Design review of the part shown in the three views and the two pictorial views. Dimensions are in mm from the part's minimum x, y and z. Coordinates: 2 decimals unless noted, no trailing zeros. Loops run counter-clockwise (first coordinate to the right, second up) from the corner with the lowest first, then second, coordinate; pieces in that order, holes last. Notation, with made-up numbers: (68.5, -29) - (101.5, -29) arc R12 ccw to (101.5, -22) - close; hole circle Ø7 at (45.5, 74). An arc over 180 degrees is marked (long way). One line per item, written item: value. Start each with the question number.
1. Take a section at B-B, the plane z = 7. State the section outline as (x, y) points.
2. Take a section at D-D, the plane x = 38. State the section outline as (y, z) points, and give its area (3 significant figures).
3. To check wall thickness, follow line 1 (Z direction, x = 43.5, y = 13.75); line 2 (X direction, y = 6.5, z = 38.5); line 3 (Y direction, x = 23.5, z = 19). State the ranges of each line that lie inside material, in increasing order. Write a range as from..to.
4. The part is to be moulded in two halves that separate along X. For the marked faces 1, 2 and 3, say which applies: released by +X, released by -X, zero draft, split by the parting line, or undercut.
5. Insertion check: pin 1 (4 mm diameter, centred on y = 7.5, z = 40, fed in from -X); pin 2 (4 mm diameter, centred on x = 30.5, z = 35, fed in from -Y); pin 3 (3 mm diameter, centred on y = 4.5, z = 31.5, fed in from +X); pin 4 (5.5 mm diameter, centred on x = 37.5, y = 3.5, fed in from -Z). Each pin has a flat end and moves straight along its axis. Give the tip position at first contact, or say it passes through.
6. Take a section at C-C, the plane x = 15. State the section outline as (y, z) points, and give its area (3 significant figures).
7. Take a section at A-A, the plane y = 5. State the section outline as (x, z) points.
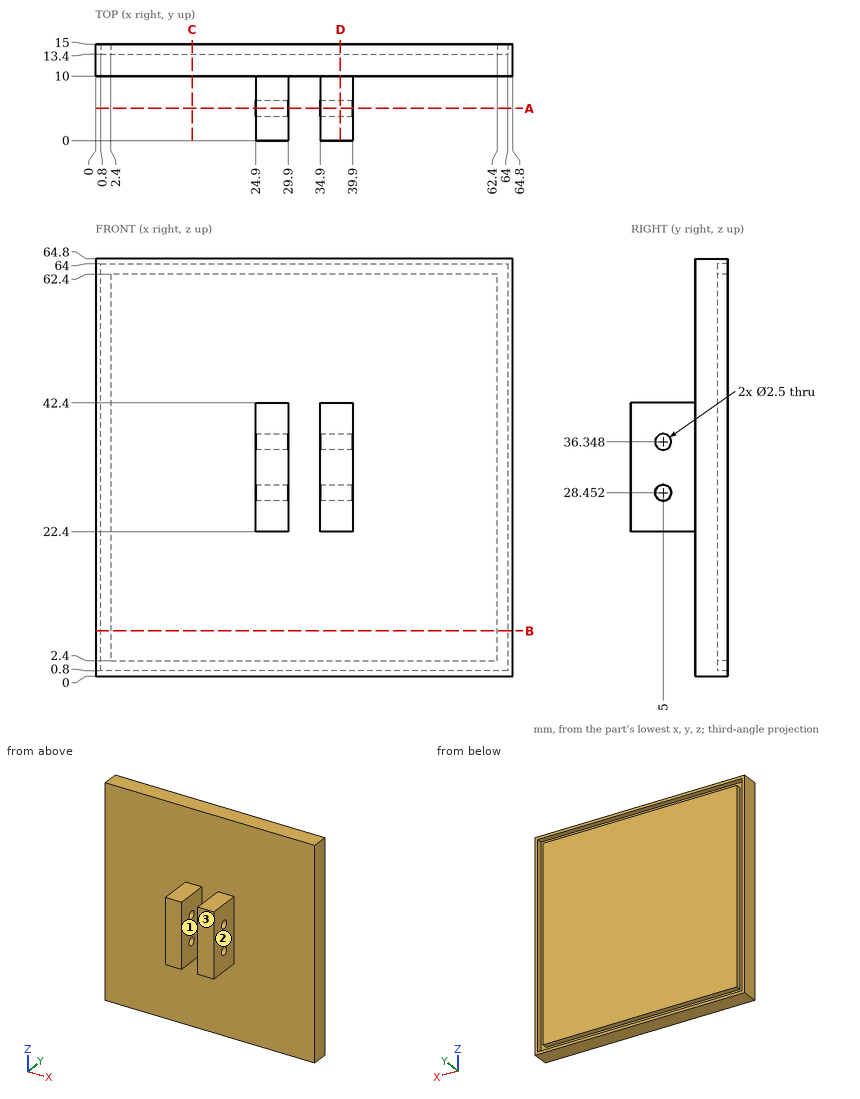
Solutions:
1. outline: (0, 10) - (64.8, 10) - (64.8, 15) - (64, 15) - (64, 13.4) - (62.4, 13.4) - (62.4, 15) - (2.4, 15) - (2.4, 13.4) - (0.8, 13.4) - (0.8, 15) - (0, 15) - close
2. outline: (0, 22.4) - (10, 22.4) - (10, 0) - (15, 0) - (15, 0.8) - (13.4, 0.8) - (13.4, 2.4) - (15, 2.4) - (15, 62.4) - (13.4, 62.4) - (13.4, 64) - (15, 64) - (15, 64.8) - (10, 64.8) - (10, 42.4) - (0, 42.4) - close; hole circle Ø2.5 at (5, 28.45); hole circle Ø2.5 at (5, 36.35)
2. area: 509 mm2
3. line 1: 0..0.8, 2.4..62.4, 64..64.8
3. line 2: 24.9..29.9, 34.9..39.9
3. line 3: 10..15
4. face 1: undercut
4. face 2: released by +X
4. face 3: zero draft
5. pin 1: x = 24.9
5. pin 2: y = 0
5. pin 3: x = 39.9
5. pin 4: z = 22.4
6. outline: (10, 0) - (15, 0) - (15, 0.8) - (13.4, 0.8) - (13.4, 2.4) - (15, 2.4) - (15, 62.4) - (13.4, 62.4) - (13.4, 64) - (15, 64) - (15, 64.8) - (10, 64.8) - close
6. area: 319 mm2
7. outline: (24.9, 22.4) - (29.9, 22.4) - (29.9, 27.2) - (24.9, 27.2) - close; (24.9, 29.7) - (29.9, 29.7) - (29.9, 35.1) - (24.9, 35.1) - close; (24.9, 37.6) - (29.9, 37.6) - (29.9, 42.4) - (24.9, 42.4) - close; (34.9, 22.4) - (39.9, 22.4) - (39.9, 27.2) - (34.9, 27.2) - close; (34.9, 29.7) - (39.9, 29.7) - (39.9, 35.1) - (34.9, 35.1) - close; (34.9, 37.6) - (39.9, 37.6) - (39.9, 42.4) - (34.9, 42.4) - close
